from build123d import *

# Parameters (mm, degrees)
F0_W     = 35
F0_H     = 5
F1_DEPTH = 1.5
F2_W     = 35
F2_H     = 1.5
F3_DEPTH = 4.5
F4_R     = 1.02
F5_DEPTH = 5.001
F6_R     = 0.5
F9_DEPTH = 35


with BuildPart() as f1:
    # F0 (on Top) → F1 (new body)
    with BuildSketch(Plane.XY):
        with Locations((17.5, -2.5)):
            Rectangle(F0_W, F0_H)
    extrude(amount=-F1_DEPTH)

    # F2 (on face) → F3 (join)
    with BuildSketch(Plane(origin=(0, 0, -1.5), x_dir=(1, 0, 0), z_dir=(0, 0, -1))):
        with Locations((17.5, 4.25)):
            Rectangle(F2_W, F2_H)
    extrude(amount=F3_DEPTH)

    # F4 (on face) → F5 (cut, through all)
    with BuildSketch(Plane.XZ.offset(5)):
        with Locations((16, -4)):
            Circle(F4_R)
    extrude(amount=-F5_DEPTH, mode=Mode.SUBTRACT)

    # F6
    f6_edges = [f1.edges().sort_by_distance(p)[0] for p in [
        (35, -4.25, -6),
        (0, -4.25, -6),
    ]]
    fillet(f6_edges, radius=F6_R)

    # F7: F1 across plane


with BuildPart() as f1_1:
    add(f1.part)
    add(f1.part.mirror(Plane.XZ))

    # F8 (on Right) → F9 (join, through all)
    with BuildSketch(Plane.YZ):
        with BuildLine():
            ThreePointArc((0, 0), (-2.522204, 0.167707), (-5, 0.667876))
            Line((-5, 0.667876), (-5, 0))
            Line((-5, 0), (0, 0))
        make_face()
        with BuildLine():
            Line((5, 0), (5, 0.667876))
            ThreePointArc((5, 0.667876), (2.522204, 0.167707), (0, 0))
            Line((0, 0), (5, 0))
        make_face()
    extrude(amount=F9_DEPTH)


solid = f1_1.part
Read the model definition and answer for the solid it produces. Units are mm, in the model's axes. A direction names the side the tool comes from. Round coordinates to 2 decimals unless told otherwise and drop trailing zeros. Loops run counter-clockwise (first coordinate to the right, second up) from the corner with the lowest first, then second, coordinate; pieces in that order, holes last.
Q1. Determine the mould class of faces 1 (the face through (35, 0, -1)), 2 (the face through (17, 4, -6)), 3 (the face through (14.98, 4.26, -3.96)) for opening direction Z: released by +Z, released by -Z, zero draft, split by the parting line, or undercut.
Q2. Section C-C on x = 16 is taken. Write down the section's boundary in (y, z), and give its area (3 significant figures).
Q3. Section A-A on z = -2 is taken. Write down the section's boundary in (x, y), and give its area (3 significant figures).
Q4. Section B-B on z = -4 is taken. Write down the section's boundary in (x, y), and give its area (3 significant figures).
Q5. Consider probe 1 along Y at (x, z) = (27.5, -2.75); probe 2 along Z at (x, y) = (16, 3.95); probe 3 along X at (y, z) = (-4, -3.5). Determine where each line is inside the solid, lowest interval first.
Q6. Each of these flat-tipped pins is pushed along its axis until it touches: pin 1 (2 mm diameter, centred on x = 15.5, y = 0.5, fed in from +Z); pin 2 (6 mm diameter, centred on x = 16.5, y = -3, fed in from +Z). Where does it stop, or does it pass through?
Q7. Which of the six approach directions +Z, -Z, +X, -X, +Y, -Y give full straight-line access (tool end or side, diameter ignored) to faces 4 (the face through (17, -5, -3)), 5 (the face through (17.3, 3.5, -3.7))?
Q8. Section D-D on x = 22.5 is taken. Write down the section's boundary in (y, z), and give its area (3 significant figures).
Output:
1. face 1: zero draft
1. face 2: released by -Z
1. face 3: undercut
2. outline: (-5, -6) - (-3.5, -6) - (-3.5, -5.02) - (-5, -5.02) - close; (-5, -2.98) - (-3.5, -2.98) - (-3.5, -1.5) - (3.5, -1.5) - (3.5, -2.98) - (5, -2.98) - (5, 0.67) arc R19.05 cw to (0, 0) arc R19.05 cw to (-5, 0.67) - close; (3.5, -6) - (5, -6) - (5, -5.02) - (3.5, -5.02) - close
2. area: 24.6 mm2
3. outline: (0, -5) - (35, -5) - (35, -3.5) - (0, -3.5) - close; (0, 3.5) - (35, 3.5) - (35, 5) - (0, 5) - close
3. area: 105 mm2
4. outline: (0, -5) - (14.98, -5) - (14.98, -3.5) - (0, -3.5) - close; (0, 3.5) - (14.98, 3.5) - (14.98, 5) - (0, 5) - close; (17.02, -5) - (35, -5) - (35, -3.5) - (17.02, -3.5) - close; (17.02, 3.5) - (35, 3.5) - (35, 5) - (17.02, 5) - close
4. area: 98.9 mm2
5. probe 1: y = -5 to -3.5, 3.5 to 5
5. probe 2: z = -6 to -5.02, -2.98 to 0.41
5. probe 3: x = 0 to 15.11, 16.89 to 35
6. pin 1: stops at z = 0.06
6. pin 2: stops at z = 0.67
7. face 4: +Z, -Z, +X, -X, -Y
7. face 5: -Z, +X, -X
8. outline: (-5, -6) - (-3.5, -6) - (-3.5, -1.5) - (3.5, -1.5) - (3.5, -6) - (5, -6) - (5, 0.67) arc R19.05 cw to (0, 0) arc R19.05 cw to (-5, 0.67) - close
8. area: 30.7 mm2
